Autodesk Inventor part; units mm, degrees
ref_plane "YZ Plane" through (0, 0, 0) normal (1, 0, 0) x (0, 1, 0)
ref_plane "XZ Plane" through (0, 0, 0) normal (0, 1, 0) x (-1, 0, 0)
ref_plane "XY Plane" through (0, 0, 0) normal (0, 0, 1) x (1, 0, 0)
sketch "Sketch1" plane through (0, 0, 0) normal (0, 1, 0) x (-1, 0, 0)
  line L0 (0, 0) -> (0, 47)
  line L1 (0, 47) -> (30, 47)
  line L2 (30, 47) -> (30, 0)
  line L3 (30, 0) -> (0, 0)
  dimension "d0" = 47
  dimension "d1" = 30
extrude "Extrusion1" add sketch "Sketch1" along normal blind 19.05
sketch "Sketch2" plane through (0, 19.05, 0) normal (0, 1, 0) x (1, 0, 0)
  line L0 (-30, 0) -> (-30, -47) construction
  line L1 (0, 0) -> (-30, 0) construction
  circle A0 centre (-25.5, -43.5) radius 1.7
  circle A1 centre (-4.5, -43.5) radius 1.7
  circle A2 centre (-23.5, -32) radius 1.7
  circle A3 centre (-6.5, -32) radius 1.7
  circle A4 centre (-23.5, -15) radius 1.7
  circle A5 centre (-25.5, -3.5) radius 1.7
  circle A6 centre (-4.5, -3.5) radius 1.7
  circle A7 centre (-6.5, -15) radius 1.7
  line L2 (-23.5, -32) -> (-23.5, -15)
  line L3 (-23.5, -15) -> (-6.5, -15)
  line L4 (-25.5, -43.5) -> (-25.5, -3.5)
  line L5 (-25.5, -3.5) -> (-4.5, -3.5)
  circle A8 centre (-15, -23.5) radius 6.25
  line L6 (-21.25, -23.5) -> (-21.25, -17.25)
  line L7 (-21.25, -17.25) -> (-8.75, -17.25)
  line L8 (-8.75, -17.25) -> (-8.75, -23.5)
  point P0 (-25.5, -23.5)
  point P1 (-30, -23.5)
  point P2 (-23.5, -23.5)
  point P3 (-30, -23.5)
  point P4 (-15, -3.5)
  point P5 (-15, 0)
  point P6 (-15, -15)
  point P7 (-15, 0)
  point P8 (-15, 0)
  point P9 (-30, -23.5)
  point P10 (-15, -17.25)
  dimension "d4" = 3.4
  dimension "d5" = 17
  dimension "d6" = 17
  dimension "d7" = 40
  dimension "d8" = 21
  dimension "d9" = 12.5
extrude "Extrusion2" cut sketch "Sketch2" against normal through all
properties part number "HopefullyHelpsMount"
Could you check a few things on this model? Use its own coordinates, in mm. A direction names the side the tool comes from. Coordinates: 2 decimals unless noted, no trailing zeros. Order: outer loops, then holes, each group sorted by start corner. A loop starts at its lowest first (then second) coordinate and runs counter-clockwise, first axis right, second up.
Q1. Suppose I cut it at B-B on y = 9.75. Give the number of separate pieces and of enclosed holes in the cut face, and give its area (3 significant figures).
Q2. Which directions (+Z, -Z, +X, -X, +Y, -Y) give clear straight access to the entire face, cutting with the end or side of a thin tool? Please do faces 1 (the cylindrical face through (-15.14, 9.66, 29.75)), 2 (the flat face through (-11, 0, 29)).
Q3. Thinking about a two-plate mould opening in X: for faces 3 (the cylindrical face through (-21.93, 9.66, 15.65)), 4 (the flat face through (-15, 9, 47)), 5 (the flat face through (0, 9, 23)), which applies, released by +X, released by -X, zero draft, split by the parting line, or undercut?
Q4. Suppose I cut it at C-C on z = 3.5. Please give me the cut outline in (x, y).
Q5. Suppose I cut it at A-A on z = 18.5. Please give me the cut outline in (x, y).
Q6. Please list where these lines run through material, in increasing order: L1, parallel to Z at x = -25.5, y = 14.75; L2, parallel to Z at x = -6.5, y = 6.5; L3, parallel to X at y = 5.5, z = 32.
Q7. Will this pin go through, and if not, where does the flat tip stop? pin 1 (6 mm diameter, centred on x = -22, z = 41.5, fed in from -Y).
Q8. Suppose I cut it at D-D on x = -16.5. Please give me the cut outline in (y, z), and give its area (3 significant figures).
Answer:
1. separate pieces: 1
1. enclosed holes: 9
1. area: 1,200 mm2
2. face 1: +Y, -Y
2. face 2: +Z, -Z, +X, -X, -Y
3. face 3: undercut
3. face 4: zero draft
3. face 5: released by +X
4. outline: (-30, 0) - (-27.2, 0) - (-27.2, 19.05) - (-30, 19.05) - close; (-23.8, 0) - (-6.2, 0) - (-6.2, 19.05) - (-23.8, 19.05) - close; (-2.8, 0) - (0, 0) - (0, 19.05) - (-2.8, 19.05) - close
5. outline: (-30, 0) - (-21.25, 0) - (-21.25, 19.05) - (-30, 19.05) - close; (-8.75, 0) - (0, 0) - (0, 19.05) - (-8.75, 19.05) - close
6. L1: z = 0 to 1.8, 5.2 to 41.8, 45.2 to 47
6. L2: z = 0 to 13.3, 16.7 to 30.3, 33.7 to 47
6. L3: x = -30 to -25.2, -21.8 to -8.2, -4.8 to 0
7. pin 1: stops at y = 0
8. outline: (0, 0) - (19.05, 0) - (19.05, 17.25) - (0, 17.25) - close; (0, 29.57) - (19.05, 29.57) - (19.05, 47) - (0, 47) - close
8. area: 661 mm2
